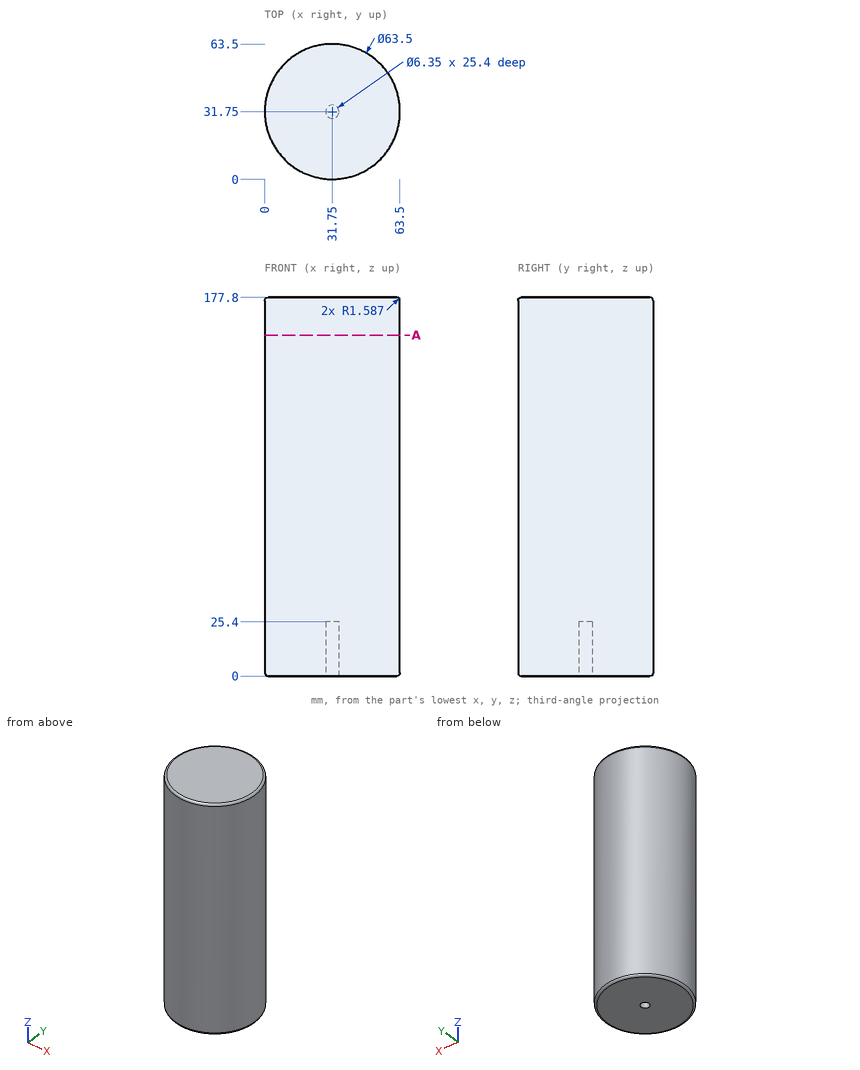
Answer from the drawing. Dimensions are ordinates in mm from the lowest x, y and z of the part. Give positions to 0.01 mm unless a question says otherwise; leave off trailing zeros. Order: outer loops, then holes, each group sorted by start corner. A loop starts at its lowest first (then second) coordinate and runs counter-clockwise, first axis right, second up. Notation, with made-up numbers: (-24, 83) -> (-17, 83) arc R24 ccw to (-17, 122) -> close; hole circle Ø6 at (1, 9). An arc over 180 degrees is marked (long way). One line per item, written item: value. Start each with the question number.
(1) Flat-ended cylindrical pins translate along their axes: P1, Ø1, axis at x = 34.5, z = 146, coming from the -Y side; P2, Ø2, axis at y = 28.5, z = 92.5, coming from the +X side; P3, Ø5, axis at x = 34, z = 135, coming from the -Y side. Find the tip coordinate at first contact, or state that the pin passes through.
(2) The part is cut by section A-A (z = 160). Determine the outline of the cut face in (x, y).
(3) Straight lines are drawn through the part: L1, parallel to Y at x = 31.75, z = 8.25 (1 decimal); L2, parallel to X at y = 31.5, z = 162; L3, parallel to Y at x = 31, z = 8 (1 decimal). For each, find the intervals that lie inside material, in ascending order.
Taken from the geometry:
1. P1: y = 0.08
1. P2: x = 63.42
1. P3: y = 0
2. outline: circle Ø63.5 at (31.75, 31.75)
3. L1: 0 to 28.6, 34.9 to 63.5
3. L2: 0 to 63.5
3. L3: 0 to 28.7, 34.8 to 63.5
